```python
from build123d import *

# Parameters (mm, degrees)
F1_DEPTH = 63.5
F2_DEPTH = 25.4
F3_DEPTH = 7.9375
F5_R     = 5.08


with BuildPart() as f1:
    # F0 (on Front) → F1 (new body, symmetric)
    with BuildSketch(Plane.XZ):
        Polygon((-41.275, 9.525), (-41.275, -9.525), (41.275, -9.525), (41.275, 9.525), (22.225, 9.525), align=None)
    extrude(amount=F1_DEPTH, both=True)

    # F0 (on Front) → F2 (join, symmetric)
    with BuildSketch(Plane.XZ):
        with BuildLine():
            Line((22.225, 9.525), (41.275, 9.525))
            Line((41.275, 9.525), (41.275, 27.0002))
            ThreePointArc((41.275, 27.0002), (45.9246798487, 38.2255201513), (57.15, 42.8752))
            Line((57.15, 42.8752), (60.325, 42.8752))
            Line((60.325, 42.8752), (60.325, 61.9252))
            Line((60.325, 61.9252), (57.15, 61.9252))
            ThreePointArc((57.15, 61.9252), (32.4542956671, 51.6959043329), (22.225, 27.0002))
            Line((22.225, 27.0002), (22.225, 9.525))
        make_face()
        Polygon((60.325, 66.675), (60.325, 61.9252), (60.325, 42.8752), (60.325, 38.1), (85.725, 38.1), (85.3455588222, 66.675), align=None)
    extrude(amount=F2_DEPTH, both=True)

    # F0 (on Front) → F3 (join, symmetric)
    with BuildSketch(Plane.XZ):
        with BuildLine():
            add(Edge.make_bspline(
                [(-41.275, 9.525), (-40.1354804635, 41.2887968123), (11.0718579963, 62.0485283434), (57.15, 61.9252)],
                knots=[0, 0, 0, 0, 111.5045361635, 111.5045361635, 111.5045361635, 111.5045361635], degree=3))
            Line((-41.275, 9.525), (22.225, 9.525))
            Line((22.225, 9.525), (22.225, 27.0002))
            ThreePointArc((22.225, 27.0002), (32.4542956671, 51.6959043329), (57.15, 61.9252))
        make_face()
    extrude(amount=F3_DEPTH, both=True)

    # F0 (on Front) → F4 (revolve)
    with BuildSketch(Plane.XZ):
        Polygon((111.125, 66.675), (85.3455588222, 66.675), (85.725, 38.1), (111.125, 38.1), align=None)
    revolve(axis=Axis((85.5352794111, 0, 52.3875), (-0.0132776108, 0, 0.9999118486)))

    # F5
    f5_edges = [f1.edges().sort_by_distance(p)[0] for p in [
        (41.275, -63.5, 0),
        (41.275, 63.5, 0),
        (-41.275, 63.5, 0),
        (-41.275, -63.5, 0),
    ]]
    fillet(f5_edges, radius=F5_R)


solid = f1.part
```
Geometry check sheet. Reference: the model listing, model coordinates, mm. A direction names the side the tool comes from. Give positions to 0.01 mm unless a question says otherwise; leave off trailing zeros. Write each loop counter-clockwise with the first axis right and the second up, starting at its lowest first coordinate (ties: lowest second). Pieces come first, ordered by that corner, then holes.
1) Section check B-B, the plane y = -38. Record the boundary of the cut face in (x, z) (3 decimals).
2) Section check A-A, the plane z = 7. Record the boundary of the cut face in (x, y) (3 decimals), and give its area (3 significant figures).
3) Release check for a two-part mould opening along X. For faces 1 (the cylindrical face through (-39.75, 62.05, -0.13)), 2 (the flat face through (53, 25.4, 45)), 3 (the flat face through (66, -20, 38.1)) record: pulls with the +X half, pulls with the -X half, needs draft (parallel to the pull), parting line crosses it, or undercut.
4) Gauge pin test, flat ends, axial feed: pin 1 (8 mm diameter, centred on x = 12.5, z = 35.5, fed in from -Y); pin 2 (8.5 mm diameter, centred on y = -14.5, z = 16, fed in from -X) (3 decimals); pin 3 (20 mm diameter, centred on x = 72.5, y = 9.5, fed in from -Z). Record the tip position at first contact, or that the pin passes through.
5) Material ranges on L1, parallel to Y at x = 65, z = 43; L2, parallel to X at y = 21, z = 11 (3 decimals); L3, parallel to Y at x = 1, z = 37, recorded low to high.
6) Access from +Z, -Z, +X, -X, +Y, -Y to the whole of each face (thin tool, end or side, straight path). Record for faces 4 (the flat face through (-2, -7.938, 30)), 5 (the conical face through (84.465, -0.967, 38.062)).
Computed:
1. outline: (-41.275, -9.525) - (41.275, -9.525) - (41.275, 9.525) - (-41.275, 9.525) - close
2. outline: (-41.275, -58.42) arc R5.08 ccw to (-36.195, -63.5) - (36.195, -63.5) arc R5.08 ccw to (41.275, -58.42) - (41.275, 58.42) arc R5.08 ccw to (36.195, 63.5) - (-36.195, 63.5) arc R5.08 ccw to (-41.275, 58.42) - close
2. area: 10,500 mm2
3. face 1: pulls with the -X half
3. face 2: needs draft
3. face 3: undercut
4. pin 1: stops at y = -7.94
4. pin 2: stops at x = 22.225
4. pin 3: stops at z = 37.45
5. L1: y = -25.4 to 25.4
5. L2: x = 22.225 to 41.275
5. L3: y = -7.94 to 7.94
6. face 4: +Z, -X, -Y
6. face 5: -Z, +X
